Can you work these out from the model? Positions are in its coordinate system, mm. A direction names the side the tool comes from. Give positions to 0.01 mm unless a question says otherwise; leave off trailing zeros. Order: outer loops, then holes, each group sorted by start corner. A loop starts at its lowest first (then second) coordinate and runs counter-clockwise, first axis right, second up. Notation, with made-up numbers: M -17,-7.5 L 42,-7.5 A24 ccw 42,9.5 Z; hole C -6,-16.75 d8. An arc over 180 degrees is marked long. One line per question, with ' | ' between items. Start each with the question number.
1) Thinking about a two-plate mould opening in X: for faces 1 (the cylindrical face through (38, 44, 10)), 2 (the flat face through (35.5, -1, 12)), 3 (the cylindrical face through (-39, -43, 10)), which applies, +X half, -X half, draft (parallel to the pull), parting line (faces both ways), or undercut?
2) If we section it at B-B, the plane x = 8.5: Please give me the cut outline in (y, z), plus the area to 3 significant figures.
3) If we section it at D-D, the plane x = -26: Please give me the cut outline in (y, z).
4) For faces 4 (the flat face through (0, 45, 10)), 5 (the flat face through (20.5, 43, 12)), 6 (the flat face through (-35.5, -1, 12)), which set-ups out of +Z, -Z, +X, -X, +Y, -Y let a thin tool reach every point of the face, with its end or its side?
5) I'm going to push flat-ended pins straight in: pin 1 Ø4 at (x, y) = (21, -7.5) entering from +Z; pin 2 Ø3.5 at (y, z) = (43, 13.5) entering from +X; pin 3 Ø1 at (y, z) = (43.5, 9) entering from -X. Where does each tip first touch, or does it pass through?
6) If we section it at C-C, the plane y = -28.5: Please give me the cut outline in (x, z), plus the area to 3 significant figures.
7) Please list where these lines run through material, in increasing order: line 1 along Y through (x, z) = (-21.5, 4.25); line 2 along X through (y, z) = (34, 19); line 3 along Z through (x, y) = (-35, -15.5). Write a range as [from, to].
8) If we section it at A-A, the plane z = 11: Please give me the cut outline in (x, y), plus the area to 3 significant figures.
```python
from build123d import *

# Parameters (mm, degrees)
F0_W     = 80
F0_H     = 90
F1_DEPTH = 20
F2_W     = 71
F2_H     = 83.6
F3_DEPTH = 17
F4_W     = 16
F4_H     = 3.2
F5_DEPTH = 17
F6_R     = 5
F7_R     = 5


with BuildPart() as f1:
    # F0 (on Top) → F1 (new body)
    with BuildSketch(Plane.XY):
        Rectangle(F0_W, F0_H)
    extrude(amount=F1_DEPTH)

    # F2 (on face) → F3 (cut)
    with BuildSketch(Plane.XY.offset(20)):
        Rectangle(F2_W, F2_H)
    extrude(amount=-F3_DEPTH, mode=Mode.SUBTRACT)

    # F4 (on face) → F5 (cut, through all)
    with BuildSketch(Plane.XY.offset(20)):
        with Locations((12.5, 43.4)):
            Rectangle(F4_W, F4_H)
    extrude(amount=-F5_DEPTH, mode=Mode.SUBTRACT)

    # F6
    f6_edges = [f1.edges().sort_by_distance(p)[0] for p in [
        (40, 45, 10),
        (40, -45, 10),
        (-40, -45, 10),
        (-40, 45, 10),
    ]]
    fillet(f6_edges, radius=F6_R)

    # F7
    f7_edges = [f1.edges().sort_by_distance(p)[0] for p in [
        (35.5, -41.8, 11.5),
        (35.5, 41.8, 11.5),
        (-35.5, 41.8, 11.5),
        (-35.5, -41.8, 11.5),
    ]]
    fillet(f7_edges, radius=F7_R)


solid = f1.part
```
Results found:
1) face 1: +X half | face 2: undercut | face 3: -X half
2) outline: M -45,0 L 45,0 L 45,3 L -41.8,3 L -41.8,20 L -45,20 Z | area: 324 mm²
3) outline: M -45,0 L 45,0 L 45,20 L 41.8,20 L 41.8,3 L -41.8,3 L -41.8,20 L -45,20 Z
4) face 4: +Z, -Z, +X, -X, +Y | face 5: +Z, +Y | face 6: +Z
5) pin 1: stops at z = 3 | pin 2: stops at x = 39.84 | pin 3: stops at x = -39
6) outline: M -40,0 L 40,0 L 40,20 L 35.5,20 L 35.5,3 L -35.5,3 L -35.5,20 L -40,20 Z | area: 393 mm²
7) line 1: y = [-45, -41.8], [41.8, 45] | line 2: x = [-40, -35.5], [35.5, 40] | line 3: z = [0, 3]
8) outline: M -40,-40 A5 ccw -35,-45 L 35,-45 A5 ccw 40,-40 L 40,40 A5 ccw 35,45 L 20.5,45 L 20.5,41.8 L 30.5,41.8 A5 cw 35.5,36.8 L 35.5,-36.8 A5 cw 30.5,-41.8 L -30.5,-41.8 A5 cw -35.5,-36.8 L -35.5,36.8 A5 cw -30.5,41.8 L 4.5,41.8 L 4.5,45 L -35,45 A5 ccw -40,40 Z | area: 1,210 mm²
